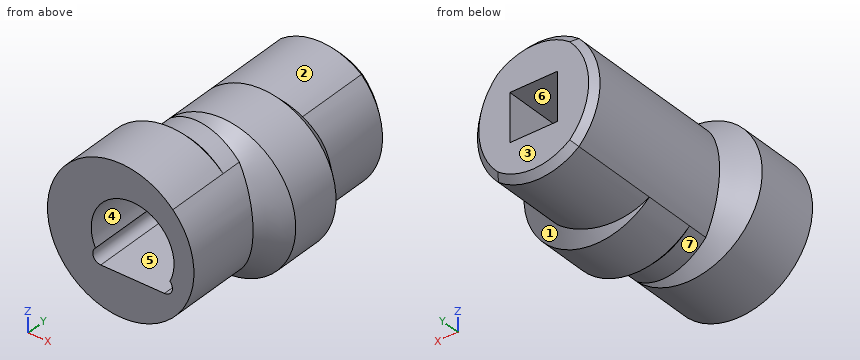
```python
from build123d import *

# Parameters (mm, degrees)
BOSS_EXTRUDE1_DEPTH = 15.4
CUT_EXTRUDE1_DEPTH  = 9.4
CUT_EXTRUDE2_REACH  = 18.939
SKETCH5_W           = 3
SKETCH5_H           = 3
CHAMFER1_SIZE       = 0.4


with BuildPart() as part:
    # Sketch1 → Boss-Extrude1 (new body)
    with BuildSketch(Plane(origin=(0, 0, 0), x_dir=(1, 0, 0), z_dir=(0, 1, 0))):
        with BuildLine():
            ThreePointArc((-2.525, -3.23022832), (0, -4.1), (2.525, -3.23022832))
            ThreePointArc((2.525, -3.23022832), (3.85, 0), (2.525, 3.23022832))
            ThreePointArc((2.525, 3.23022832), (0, 4.1), (-2.525, 3.23022832))
            ThreePointArc((-2.525, 3.23022832), (-3.85, 0), (-2.525, -3.23022832))
        make_face()
    extrude(amount=BOSS_EXTRUDE1_DEPTH)

    # Sketch2 → Revolve1 (revolve)
    with BuildSketch(Plane.XY, mode=Mode.PRIVATE) as revolve1_sk:
        Polygon((3.85, 0), (3.85, 4), (2.35, 5.5), (-0.75, 5.5), (-0.75, 0), align=None)
    revolve(revolve1_sk.sketch.rotate(Axis((-0.75, 5.5, 0), (0, -1, 0)), 270), axis=Axis((-0.75, 5.5, 0), (0, -1, 0)))

    # Sketch3 → Revolve2 (revolve)
    with BuildSketch(Plane.XY, mode=Mode.PRIVATE) as revolve2_sk:
        Polygon((0.75, 4.7), (-2.35, 4.7), (-3.85, 6.2), (-3.85, 9.4), (-2.35, 10.9), (0.75, 10.9), align=None)
    revolve(revolve2_sk.sketch.rotate(Axis((0.75, 4.7, 0), (0, 1, 0)), 315.394327097), axis=Axis((0.75, 4.7, 0), (0, 1, 0)))

    # Sketch4 → Cut-Extrude1 (cut)
    with BuildSketch(Plane.XZ):
        with BuildLine():
            Line((-2, -2), (2, -2))
            ThreePointArc((2, -2), (2.465465068, -1.682598659), (2.339973189, -1.133369081))
            ThreePointArc((2.339973189, -1.133369081), (0, 2.6), (-2.339973189, -1.133369081))
            ThreePointArc((-2.339973189, -1.133369081), (-2.465465068, -1.682598659), (-2, -2))
        make_face()
    extrude(amount=-CUT_EXTRUDE1_DEPTH, mode=Mode.SUBTRACT)

    # Sketch5 → Cut-Extrude2 (cut, up to next)
    with BuildSketch(Plane(origin=(0, 15.4, 0), x_dir=(1, 0, 0), z_dir=(0, 1, 0)), mode=Mode.PRIVATE) as cut_extrude2_sk1:
        Rectangle(SKETCH5_W, SKETCH5_H)
    cut_extrude2_tool1 = extrude(cut_extrude2_sk1.sketch, amount=-CUT_EXTRUDE2_REACH, mode=Mode.PRIVATE) & part.part
    add(cut_extrude2_tool1.solids().sort_by_distance((0, 15.4, 0))[0], mode=Mode.SUBTRACT)

    # Chamfer1
    # the kernel refuses this chamfer: 0.4 mm, written as the material it takes off along each edge
    with BuildSketch(Plane(origin=(0, 15.4, 0), x_dir=(-0.7922190522423981, 0, 0.6102368173620439), z_dir=(-0.6102368173620439, 0, -0.7922190522423981))) as chamfer1_piece_1:
        Polygon((4.1 - CHAMFER1_SIZE, 0), (4.1, -CHAMFER1_SIZE), (4.1, 0), align=None)
    revolve(axis=Axis((0, 15.4, 0), (0, 1, 0)), revolution_arc=104.786743256, mode=Mode.SUBTRACT)
    with BuildSketch(Plane(origin=(-0.75, 15.4, 0), x_dir=(0.5384255548923128, 0, 0.8426730812354843), z_dir=(-0.8426730812354843, 0, 0.5384255548923128))) as chamfer1_piece_2:
        Polygon((4.6 - CHAMFER1_SIZE, 0), (4.6, -CHAMFER1_SIZE), (4.6, 0), align=None)
    revolve(axis=Axis((-0.75, 15.4, 0), (0, 1, 0)), revolution_arc=114.846952535, mode=Mode.SUBTRACT)
    with BuildSketch(Plane(origin=(0, 15.4, 0), x_dir=(0.7922190522423987, 0, -0.610236817362043), z_dir=(0.610236817362043, 0, 0.7922190522423987))) as chamfer1_piece_3:
        Polygon((4.1 - CHAMFER1_SIZE, 0), (4.1, -CHAMFER1_SIZE), (4.1, 0), align=None)
    revolve(axis=Axis((0, 15.4, 0), (0, 1, 0)), revolution_arc=104.786743256, mode=Mode.SUBTRACT)
    with BuildSketch(Plane(origin=(0.75, 15.4, 0), x_dir=(-0.5384255548923127, 0, -0.8426730812354845), z_dir=(0.8426730812354845, 0, -0.5384255548923127))) as chamfer1_piece_4:
        Polygon((4.6 - CHAMFER1_SIZE, 0), (4.6, -CHAMFER1_SIZE), (4.6, 0), align=None)
    revolve(axis=Axis((0.75, 15.4, 0), (0, 1, 0)), revolution_arc=114.846952535, mode=Mode.SUBTRACT)


solid = part.part
```
Build history of the part. All positions in model axes, mm. Face numbers are marked on the shaded views. A direction names the side the tool comes from. Round coordinates to 2 decimals unless told otherwise and drop trailing zeros. Loops run counter-clockwise (first coordinate to the right, second up) from the corner with the lowest first, then second, coordinate; pieces in that order, holes last.
Item 1: Saw through at B-B (y = 1.75). List the corners of the cut face in (x, z) (3 decimals), then the cut area to 3 significant figures.
Item 2: Saw through at A-A (z = 0). List the corners of the cut face in (x, y).
Item 3: Pin check, flat tips, straight feed: P1, Ø6, axis at x = 3, y = 3.5, coming from the +Z side; P2, Ø3, axis at x = -3, y = 5, coming from the -Z side; P3, Ø2.5, axis at x = 0.5, y = 12, coming from the +Z side. Stop position of each tip, or through.
Item 4: Drill centre lines: line 1 along X through (y, z) = (3.5, 0); line 2 along X through (y, z) = (7, -1); line 3 along Y through (x, z) = (2.5, 0.5). Where is each one in solid material? Low to high.
Item 5: Which spindle directions (+Z, -Z, +X, -X, +Y, -Y) get a long thin tool onto all of the face, cutting with end or side? Do the marked faces 5, 6 and 7. Say none if no direction does.
Item 6: Two-plate mould, pull along Z, no slides. Class the marked faces 1, 2, 3 and 4: released by +Z, released by -Z, zero draft, split by the parting line, or undercut.
Worked answers:
1. outline: circle Ø9.2 at (-0.75, 0); hole (-2.34, -1.133) arc R0.5 ccw to (-2, -2) - (2, -2) arc R0.5 ccw to (2.34, -1.133) arc R2.6 ccw (long way) to start
1. area: 46.0 mm2
2. outline: (-5.35, 0) - (-2.6, 0) - (-2.6, 9.4) - (-1.5, 9.4) - (-1.5, 15.4) - (-3.45, 15.4) - (-3.85, 15) - (-3.85, 5.5) - (-5.35, 4) - close; (1.5, 9.4) - (2.6, 9.4) - (2.6, 0) - (3.85, 0) - (3.85, 4.7) - (5.35, 6.2) - (5.35, 9.4) - (3.85, 10.9) - (3.85, 15) - (3.45, 15.4) - (1.5, 15.4) - close
3. P1: stops at z = 4.54
3. P2: stops at z = -4.46
3. P3: stops at z = 4.1
4. line 1: x = -5.35 to -2.6, 2.6 to 3.85
4. line 2: x = -3.74 to -2.4, 2.4 to 5.24
4. line 3: y = 9.4 to 15.4
5. face 5: -Y
5. face 6: +Y, -Y
5. face 7: -Z
6. face 1: split by the parting line
6. face 2: released by +Z
6. face 3: zero draft
6. face 4: undercut
